Work out the finished part from the listing and answer in its coordinate system (mm). Give positions to 0.01 mm unless a question says otherwise; leave off trailing zeros. Loops run counter-clockwise (first coordinate to the right, second up) from the corner with the lowest first, then second, coordinate; pieces in that order, holes last. Notation, with made-up numbers: M 11.25,-23 L 63.25,-23 A14 cw 63.25,-10 Z; hole C 78.25,28.5 d11. An arc over 180 degrees is marked long. Answer in a Markdown table with one row per item. Add a question column.
from build123d import *

# Parameters (mm, degrees)
F1_DEPTH    = 4
F4_D        = 3.2
F5_T1_DEPTH = 14.1810362517


# Not quite as in the source:
# - a fillet or chamfer that OpenCascade refuses, or shapes differently, is made with other operations: its cross-section is extruded or revolved along the edge and cut away or added


with BuildPart() as f1:
    # F0 (on Top) → F1 (new body)
    with BuildSketch(Plane.XY):
        with BuildLine():
            ThreePointArc((54.4209333808, 71.682368892), (73.4574706888, 52), (85.6943365292, 27.5041939859))
            Line((85.6943365292, 27.5041939859), (90.4551330031, 29.0322047629))
            ThreePointArc((90.4551330031, 29.0322047629), (77.5384412827, 54.8888888889), (57.4443185686, 75.6647227193))
            Line((57.4443185686, 75.6647227193), (54.4209333808, 71.682368892))
        make_face()
    extrude(amount=F1_DEPTH)

    # F4 (through all)
    with Locations(Plane.YZ.offset(90.457)):
        with Locations((39.0287227929, 1.9947474357), (63.0079358816, 2.0034648478)):
            Hole(F4_D / 2)

    # F5: chamfer of 2 on 2 edges, made by hand

    # F5_s2 → F5_t1 (cut)
    with BuildSketch(Plane.XY.offset(-5.0905181258)):
        with BuildLine():
            Line((87.5779535576, 28.1087539864), (85.0761677414, 29.3606144765))
            ThreePointArc((85.0761677414, 29.3606144765), (85.3813536757, 28.4609283843), (85.6943365292, 27.5041939859))
            Line((85.6943365292, 27.5041939859), (87.5779535576, 28.1087539864))
        make_face()
        with BuildLine():
            Line((55.6171407495, 73.2579937949), (55.9663848396, 70.4823649432))
            ThreePointArc((55.9663848396, 70.4823649432), (55.2192662472, 71.0692101766), (54.4209333808, 71.682368892))
            Line((54.4209333808, 71.682368892), (55.6171407495, 73.2579937949))
        make_face()
    extrude(amount=F5_T1_DEPTH, mode=Mode.SUBTRACT)


solid = f1.part
(1) Section C-C, the plane x = 69 is taken. Determine the outline of the cut face in (y, z), and give its area (3 significant figures).
(2) Consider line 1 along Y through (x, z) = (69.5, 1.9); line 2 along Y through (x, z) = (68, 1); line 3 along Y through (x, z) = (79, 2.8). Determine where each line is inside the solid, lowest interval first. Write a range as from..to.
(3) The mould has two halves that part along Y. Classify faces 1 (the face through (73.25, 52.29, 1.97)), 2 (the face through (74, 52, 0)), 3 (the face through (67.502, 64.606, 2.074)): pulls with the +Y half, pulls with the -Y half, needs draft (parallel to the pull), parting line crosses it, or undercut.
(4) Section A-A, the plane y = 40 is taken. Determine the outline of the cut face in (x, z), and give its area (3 significant figures).
(5) This flat-tipped pin is pushed along its axis until it touches: P1, Ø1, axis at y = 62.5, z = 0.5, coming from the -X side. Where does it stop, or does it pass through?
(6) Section D-D, the plane y = 63 is taken. Determine the outline of the cut face in (x, z).
(7) Section B-B, the plane z = 2.7 is taken. Determine the outline of the cut face in (x, y).
Numbers:
| question | item | result |
|---|---|---|
| 1 | outline | M 57.78,0 L 65.3,0 L 65.3,4 L 57.78,4 Z; hole C 63.01,2 d3.2 |
| 1 | area | 22.0 mm² |
| 2 | line 1 | y = 57.18..61.41, 64.6..64.77 |
| 2 | line 2 | y = 58.96..61.76, 64.25..66.34 |
| 2 | line 3 | y = 43.12..52.76 |
| 3 | face 1 | pulls with the -Y half |
| 3 | face 2 | needs draft |
| 3 | face 3 | undercut |
| 4 | outline | M 80.62,0 L 86.17,0 L 86.17,0.72 L 80.62,0.72 Z; M 80.62,3.27 L 86.17,3.27 L 86.17,4 L 80.62,4 Z |
| 4 | area | 8.08 mm² |
| 5 | P1 | stops at x = 64.28 |
| 6 | outline | M 64.27,0 L 71.11,0 L 71.11,0.4 L 64.27,0.4 Z; M 64.27,3.6 L 71.11,3.6 L 71.11,4 L 64.27,4 Z |
| 7 | outline | M 55.62,73.26 L 55.97,70.48 A90 cw 62.82,64.45 L 69.8,64.45 A95 ccw 57.44,75.66 Z; M 65.65,61.57 A90 cw 80.39,40.46 L 85.95,40.46 A95 ccw 72.35,61.57 Z; M 81.77,37.59 A90 cw 85.08,29.36 L 87.58,28.11 L 90.46,29.03 A95 ccw 87.25,37.59 Z |
